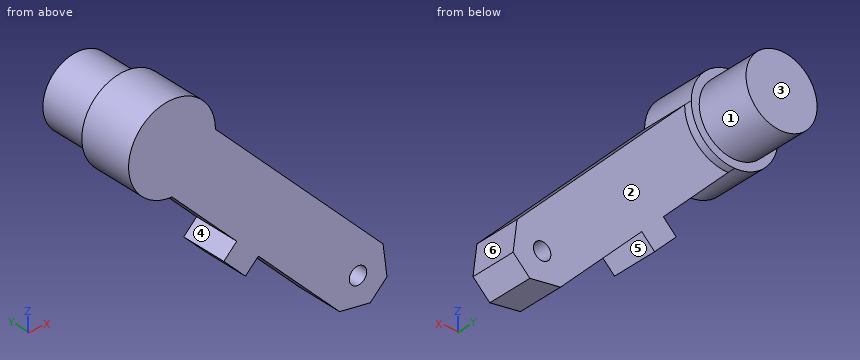
from build123d import *

# Parameters (mm, degrees)
F0_R     = 1.1
F0_R_2   = 4.5
F1_DEPTH = 6
F2_DEPTH = 1
F3_DEPTH = 8


with BuildPart() as f1:
    # F0 (on Front) → F1 (new body)
    with BuildSketch(Plane.XZ):
        with BuildLine():
            Line((26.7132034356, -21.2132034356), (5.5, 0))
            ThreePointArc((5.5, 0), (3.8890872965, -3.8890872965), (0, -5.5))
            Line((0, -5.5), (8.1949569136, -13.6949569136))
            Line((8.1949569136, -13.6949569136), (10.9329223484, -16.4329223484))
            Line((10.9329223484, -16.4329223484), (21.2132034356, -26.7132034356))
            Line((21.2132034356, -26.7132034356), (25.0945742855, -27.2313275223))
            Line((25.0945742855, -27.2313275223), (27.2158946291, -25.1100071787))
            Line((27.2158946291, -25.1100071787), (26.7132034356, -21.2132034356))
        make_face()
        with Locations((23.5389393669, -23.5543722601)):
            Circle(F0_R, mode=Mode.SUBTRACT)
        with BuildLine():
            ThreePointArc((0, -5.5), (3.8890872965, -3.8890872965), (5.5, 0))
            ThreePointArc((5.5, 0), (-3.8890872965, 3.8890872965), (0, -5.5))
        make_face()
        Circle(F0_R_2, mode=Mode.SUBTRACT)
        Circle(F0_R_2)
        Polygon((10.9329223484, -16.4329223484), (8.1949569136, -13.6949569136), (6.5603537951, -15.3295600321), (9.2983192299, -18.0675254669), align=None)
    extrude(amount=F1_DEPTH)

    # F0 (on Front) → F2 (join)
    with BuildSketch(Plane.XZ):
        with BuildLine():
            ThreePointArc((0, -5.5), (3.8890872965, -3.8890872965), (5.5, 0))
            ThreePointArc((5.5, 0), (-3.8890872965, 3.8890872965), (0, -5.5))
        make_face()
        Circle(F0_R_2, mode=Mode.SUBTRACT)
        Circle(F0_R_2)
    extrude(amount=-F2_DEPTH)

    # F0 (on Front) → F3 (join)
    with BuildSketch(Plane.XZ):
        Circle(F0_R_2)
    extrude(amount=-F3_DEPTH)


solid = f1.part
Geometry: final body of the model. Coordinates: model frame, mm. Face numbers are marked on the shaded views. A direction names the side the tool comes from. Give positions to 0.01 mm unless a question says otherwise; leave off trailing zeros. Order: outer loops, then holes, each group sorted by start corner. A loop starts at its lowest first (then second) coordinate and runs counter-clockwise, first axis right, second up. Notation, with made-up numbers: (44, 30.5) -> (85, 30.5) arc R17 cw to (85, 60.5) -> close; hole circle Ø9 at (57, -27.75). An arc over 180 degrees is marked (long way). Answer as a JSON object with one key per item and string values.
Q1. Material intervals for probe 1 along Y at (x, z) = (21, -19.5); probe 2 along X at (y, z) = (-2.75, -24.5); probe 3 along X at (y, z) = (4.25, 1), sorted ascending.
Entries:
{"probe 1": "y = -6 to 0", "probe 2": "x = 19 to 22.98, 24.1 to 27.14", "probe 3": "x = -4.39 to 4.39"}
Q2. Draft query along X for the marked faces 4, 5 and 6. Return one class per face: released by +X, released by -X, zero draft, split by the parting line, or undercut.
Entries:
{"face 4": "released by -X", "face 5": "undercut", "face 6": "released by +X"}
Q3. Access query for the marked faces 1, 2 and 3. Directions: +Z, -Z, +X, -X, +Y, -Y. A direction counts if a zero-diameter tool reaches every point of the face in a straight line with its end or side. Return the directions, or none.
Entries:
{"face 1": "+Y", "face 2": "-Z, +X, +Y", "face 3": "+Z, -Z, +X, -X, +Y"}
Q4. Section A-A (x = 24). Output: boundary loops of the cut face in (y, z), plus the area to 3 significant figures.
Entries:
{"outline": "(-6, -27.09) -> (0, -27.09) -> (0, -24.55) -> (-6, -24.55) -> close; (-6, -22.56) -> (0, -22.56) -> (0, -18.5) -> (-6, -18.5) -> close", "area": "39.5 mm^2"}
Q5. First-contact query: pin 1 (3 mm diameter, centred on x = 12, z = -9, fed in from +Y); pin 2 (5 mm diameter, centred on x = 20.5, z = -8, fed in from -Y); pin 3 (2 mm diameter, centred on y = 0.5, z = -20, fed in from -X); pin 4 (3 mm diameter, centred on x = 1, y = 0.5, fed in from -Z). Flat tips, straight axial feed; report the tip coordinate or a pass-through.
Entries:
{"pin 1": "stops at y = 0", "pin 2": "passes through", "pin 3": "stops at x = 13.63", "pin 4": "stops at z = -7.91"}
Q6. Section C-C (y = -4.5). Output: boundary loops of the cut face in (x, z), plus the area to 3 significant figures.
Entries:
{"outline": "(0, -5.5) -> (8.19, -13.69) -> (6.56, -15.33) -> (9.3, -18.07) -> (10.93, -16.43) -> (21.21, -26.71) -> (25.09, -27.23) -> (27.22, -25.11) -> (26.71, -21.21) -> (5.5, 0) arc R5.5 ccw (long way) to start; hole circle Ø2.2 at (23.54, -23.55)", "area": "342 mm^2"}
Q7. Section D-D (x = -3). Output: boundary loops of the cut face in (y, z).
Entries:
{"outline": "(-6, -4.61) -> (1, -4.61) -> (1, -3.35) -> (8, -3.35) -> (8, 3.35) -> (1, 3.35) -> (1, 4.61) -> (-6, 4.61) -> close"}
Q8. Section B-B (z = -23). Output: boundary loops of the cut face in (x, y).
Entries:
{"outline": "(17.5, -6) -> (22.59, -6) -> (22.59, 0) -> (17.5, 0) -> close; (24.49, -6) -> (26.94, -6) -> (26.94, 0) -> (24.49, 0) -> close"}
